Can you work these out from the model? Positions are in its coordinate system, mm. A direction names the side the tool comes from. Give positions to 0.01 mm unless a question says otherwise; leave off trailing zeros. Loops run counter-clockwise (first coordinate to the right, second up) from the corner with the lowest first, then second, coordinate; pieces in that order, holes last. Notation, with made-up numbers: (-8.75, -0.75) -> (-3.75, -0.75) arc R14 cw to (-3.75, 16.25) -> close; hole circle Ø2 at (-24, 52.25). An arc over 180 degrees is marked (long way). Use CSV: the item, a comma, the result in double quotes.
from build123d import *

# Parameters (mm, degrees)
F1_DEPTH = 24


with BuildPart() as f1:
    # F0 (on Top) → F1 (new body)
    with BuildSketch(Plane.XY):
        with BuildLine():
            Line((-131, 0), (0, 0))
            Line((0, 0), (0, 762))
            Line((0, 762), (-643, 762))
            ThreePointArc((-643, 762), (-996.553391, 615.553391), (-1143, 262))
            Line((-1143, 262), (-1143, -381))
            Line((-1143, -381), (-381, -381))
            Line((-381, -381), (-381, -250))
            ThreePointArc((-381, -250), (-307.776695, -73.223305), (-131, 0))
        make_face()
    extrude(amount=F1_DEPTH)

    # F4: sweep along a path in F3
    with BuildLine(Plane(origin=(0, 0, 0), x_dir=(1, 0, 0), z_dir=(0, 0, -1))) as f4_path:
        Line((0, 0), (-131, 0))
        ThreePointArc((-131, 0), (-307.776695, 73.223305), (-381, 250))
        Line((-381, 250), (-381, 381))
    # F2 (on face) → F4 (sweep, cut)
    with BuildSketch(Plane.YZ):
        Polygon((0, 0), (50, 0), (0, 14), align=None)
    sweep(path=f4_path.line, mode=Mode.SUBTRACT)

    # F5: sweep along a path in F3
    with BuildLine(Plane(origin=(0, 0, 0), x_dir=(1, 0, 0), z_dir=(0, 0, -1))) as f5_path:
        Line((0, -762), (-643, -762))
        ThreePointArc((-643, -762), (-996.553391, -615.553391), (-1143, -262))
        Line((-1143, -262), (-1143, 381))
    # F2 (on face) → F5 (sweep, cut)
    with BuildSketch(Plane.YZ):
        Polygon((762, 0), (762, 14), (712, 0), align=None)
    sweep(path=f5_path.line, mode=Mode.SUBTRACT)


solid = f1.part
(1) Will these pins go through, and if not, where does the flat tip stop? pin 1 Ø10 at (x, y) = (-727.5, -100) entering from -Z; pin 2 Ø3 at (x, z) = (-97.5, 19.5) entering from -Y; pin 3 Ø3 at (y, z) = (-315.5, 18) entering from +X.
Answer sheet:
pin 1,"stops at z = 0"
pin 2,"stops at y = 0"
pin 3,"stops at x = -381"
(2) We'd pull the mould along Y, two halves only. Please class faces 3 (the face through (-959.38, 585.41, 0.68)), 4 (the face through (-406, -316, 7)), 5 (the face through (-309.71, -75.18, 18.93)): released by +Y, released by -Y, zero draft, split by the parting line, or undercut.
Answer sheet:
face 3,"released by +Y"
face 4,"zero draft"
face 5,"released by -Y"
(3) If I drill on L1, parallel to X at y = -241, z = 16.5; L2, parallel to Y at x = -893.5, z = 15; L3, parallel to X at y = 625, z = 15.5, over which ranges is the centre line in solid material (lowest first)? Write a range as from..to.
Answer sheet:
L1,"x = -1143..-380.84"
L2,"y = -381..694.72"
L3,"x = -986.85..0"
(4) If we section it at A-A, the plane z = 19.5: Write out the boundary of the cut face in (x, y), then the cut area to 3 significant figures.
Answer sheet:
outline,"(-1143, -381) -> (-381, -381) -> (-381, -250) arc R250 cw to (-131, 0) -> (0, 0) -> (0, 762) -> (-643, 762) arc R500 ccw to (-1143, 262) -> close"
area,"1,120,000 mm2"
(5) If we section it at B-B, the plane y = -301: Write out the boundary of the cut face in (x, z).
Answer sheet:
outline,"(-1143, 14) -> (-1093, 0) -> (-431, 0) -> (-381, 14) -> (-381, 24) -> (-1143, 24) -> close"
(6) Which directions (+Z, -Z, +X, -X, +Y, -Y) give clear straight access to the entire face, cutting with the end or side of a thin tool? Please do faces 1 (the face through (-66, 25, 7)), 2 (the face through (-1118, -64, 7)).
Answer sheet:
face 1,"-Z, +X, -Y"
face 2,"-Z, -X, +Y, -Y"
